```python
from build123d import *

# Parameters (mm, degrees)
EXTRUDE_1_DEPTH       = 30
HOLE_WIZARD_3_0_3_1_D = 3


with BuildPart() as part:
    # Эскиз1 → Бобышка-Вытянуть1 (new body)
    with BuildSketch(Plane.XY):
        Polygon((4, 0.5), (-5, 0.5), (-5, -0.5), (5, -0.5), (5, 0.5), (5, 9.5), (4, 9.5), align=None)
    extrude(amount=EXTRUDE_1_DEPTH)

    # Диаметр отверстия Ø3.0 (3)1 (through all)
    with Locations(Plane(origin=(0, 0.5, 0), x_dir=(1, 0, 0), z_dir=(0, 1, 0))):
        with Locations((-0.5, -10), (-0.5, -20)):
            Hole(HOLE_WIZARD_3_0_3_1_D / 2)


solid = part.part
```
Source: CAD feature listing. Evaluate the final solid. Frame: model axes, mm. A direction names the side the tool comes from. Give positions to 0.01 mm unless a question says otherwise; leave off trailing zeros. Write each loop counter-clockwise with the first axis right and the second up, starting at its lowest first coordinate (ties: lowest second). Pieces come first, ordered by that corner, then holes. Notation, with made-up numbers: (59, 64.25) - (98, 64.25) arc R17 ccw to (98, 77.25) - close; hole circle Ø1 at (-32.75, -2.75). An arc over 180 degrees is marked (long way). One line per item, written item: value. Start each with the question number.
Q1. Section query D-D, the plane x = -2.5. Return the cut outline in (y, z).
Q2. Section query B-B, the plane z = 10. Return the cut outline in (x, y).
Q3. Section query C-C, the plane z = 5.5. Return the cut outline in (x, y), then the cut area to 3 significant figures.
Q4. Section query A-A, the plane x = -0.5. Return the cut outline in (y, z).
Q5. Set-up query: faces 1 (the face through (0, 0.5, 15)), 2 (the face through (2, 0, 30)). Return all of +Z, -Z, +X, -X, +Y, -Y with unobstructed straight access to the full face (end or side cutting, diameter ignored); none if empty.
Q6. First-contact query: pin 1 Ø2.5 at (x, z) = (-0.5, 20) entering from +Y; pin 2 Ø4 at (y, z) = (8, 15) entering from -X; pin 3 Ø5 at (x, z) = (0.5, 8) entering from +Y. Flat tips, straight axial feed; report the tip coordinate or a pass-through.
Q7. Material intervals for probe 1 along Z at (x, y) = (-0.5, 0.1); probe 2 along Y at (x, z) = (3.25, 16.75); probe 3 along X at (y, z) = (-0.2, 20), sorted ascending. Write a range as from..to.
Q8. Draft query along X for faces 3 (the face through (5, 4, 15)), 4 (the face through (-0.175, -0.007, 11.464)), 5 (the face through (-0.305, -0.007, 18.513)), 6 (the face through (4.5, 9.5, 14.8)). Return one class per face: +X half, -X half, draft (parallel to the pull), parting line (faces both ways), or undercut.
Answer:
1. outline: (-0.5, 0) - (0.5, 0) - (0.5, 30) - (-0.5, 30) - close
2. outline: (-5, -0.5) - (-2, -0.5) - (-2, 0.5) - (-5, 0.5) - close; (1, -0.5) - (5, -0.5) - (5, 9.5) - (4, 9.5) - (4, 0.5) - (1, 0.5) - close
3. outline: (-5, -0.5) - (5, -0.5) - (5, 9.5) - (4, 9.5) - (4, 0.5) - (-5, 0.5) - close
3. area: 19.0 mm2
4. outline: (-0.5, 0) - (0.5, 0) - (0.5, 8.5) - (-0.5, 8.5) - close; (-0.5, 11.5) - (0.5, 11.5) - (0.5, 18.5) - (-0.5, 18.5) - close; (-0.5, 21.5) - (0.5, 21.5) - (0.5, 30) - (-0.5, 30) - close
5. face 1: +Z, -Z, -X, +Y
5. face 2: +Z, +X, -X, +Y, -Y
6. pin 1: passes through
6. pin 2: stops at x = 4
6. pin 3: stops at y = 0.5
7. probe 1: z = 0..8.5, 11.5..18.5, 21.5..30
7. probe 2: y = -0.5..0.5
7. probe 3: x = -5..-2, 1..5
8. face 3: +X half
8. face 4: undercut
8. face 5: undercut
8. face 6: draft
